```python
from build123d import *

# Parameters (mm, degrees)
SKETCH1_R           = 104.775
BOSS_EXTRUDE1_DEPTH = 38.1
BOSS_EXTRUDE1_DRAFT = -7.5
SKETCH2_R           = 14.2875
CUT_EXTRUDE1_DEPTH  = 153.9941543
SKETCH3_R           = 3.175
CUT_EXTRUDE2_DEPTH  = 38.1


with BuildPart() as part:
    # Sketch1 → Boss-Extrude1 (with draft: the straight prism first)
    with BuildSketch(Plane.XY):
        Circle(SKETCH1_R)
    extrude(amount=-BOSS_EXTRUDE1_DEPTH)
    # Boss-Extrude1: the draft: its side faces are tilted about the plane it starts from
    boss_extrude1_sides = [part.faces().sort_by_distance(p)[0] for p in [
        (-104.775, 0, -19.05),
    ]]
    draft(boss_extrude1_sides, Plane.XY, BOSS_EXTRUDE1_DRAFT)

    # Sketch2 → Cut-Extrude1 (cut, through all)
    with BuildSketch(Plane.XY):
        Circle(SKETCH2_R)
    extrude(amount=-CUT_EXTRUDE1_DEPTH, mode=Mode.SUBTRACT)

    # Sketch3 → Cut-Extrude2 (cut)
    with BuildSketch(Plane.XY):
        with Locations((34.925, 0)):
            Circle(SKETCH3_R)
        with Locations((17.4625, -30.245937227)):
            Circle(SKETCH3_R)
        with Locations((-17.4625, -30.245937227)):
            Circle(SKETCH3_R)
        with Locations((-34.925, 0)):
            Circle(SKETCH3_R)
        with Locations((-17.4625, 30.245937227)):
            Circle(SKETCH3_R)
        with Locations((17.4625, 30.245937227)):
            Circle(SKETCH3_R)
    extrude(amount=-CUT_EXTRUDE2_DEPTH, mode=Mode.SUBTRACT)


solid = part.part
```
For this review, take the finished solid that the model builds, in its own axes (mm). Round coordinates to 2 decimals unless told otherwise and drop trailing zeros. Write each loop counter-clockwise with the first axis right and the second up, starting at its lowest first coordinate (ties: lowest second). Pieces come first, ordered by that corner, then holes. Notation, with made-up numbers: (-13.5, -25.5) -> (35.5, -25.5) arc R17 cw to (35.5, -20.5) -> close; hole circle Ø8 at (51, 29.5). An arc over 180 degrees is marked (long way). One line per question, with ' | ' between items. Start each with the question number.
(1) Insertion check: P1, Ø5.5, axis at x = 17.46, y = -30.25, coming from the -Z side; P2, Ø1, axis at x = -43.5, z = -21.5, coming from the -Y side; P3, Ø8, axis at y = -26.5, z = -24, coming from the +X side; P4, Ø1.5, axis at x = -56.5, z = -32.5, coming from the +Y side. Each pin has a flat end and moves straight along its axis. Give the tip position at first contact, or say it passes through.
(2) Add section B-B, the plane x = 0. Write out the cut boundary in (y, z) (1 decimal), plus the area to 3 significant figures.
(3) For line 1 along X through (y, z) = (1, -27); line 2 along X through (y, z) = (2.5, -28); line 3 along Y through (x, z) = (-13, -10.5), list the stretches that pass through material, from the lowest coordinate up. Write a range as from..to.
(4) Mouldability with a two-part tool opening along X and no side actions: class faces 1 (the face through (-1, -22, 0)), 2 (the face through (95.983, 30.227, -31.483)), 3 (the face through (20.395, 29.03, -18.783)), 4 (the face through (-18.151, 27.146, -18.783)) as released by +X, released by -X, zero draft, split by the parting line, or undercut.
(5) Add section A-A, the plane y = 0. Give the number of separate pieces and of enclosed holes in the cut face, plus the area to 3 significant figures.
Answer list:
1) P1: through | P2: y = -92.44 | P3: x = 99.24 | P4: y = 83.63
2) outline: (-104.8, 0) -> (-99.8, -38.1) -> (-14.3, -38.1) -> (-14.3, 0) -> close; (14.3, -38.1) -> (99.8, -38.1) -> (104.8, 0) -> (14.3, 0) -> close | area: 6,700 mm²
3) line 1: -101.22..-37.94, -31.91..-14.25, 14.25..31.91, 37.94..101.22 | line 2: -101.06..-36.88, -32.97..-14.07, 14.07..32.97, 36.88..101.06 | line 3: -102.57..-5.93, 5.93..102.57
4) face 1: zero draft | face 2: split by the parting line | face 3: undercut | face 4: undercut
5) separate pieces: 4 | enclosed holes: 0 | area: 6,220 mm²
